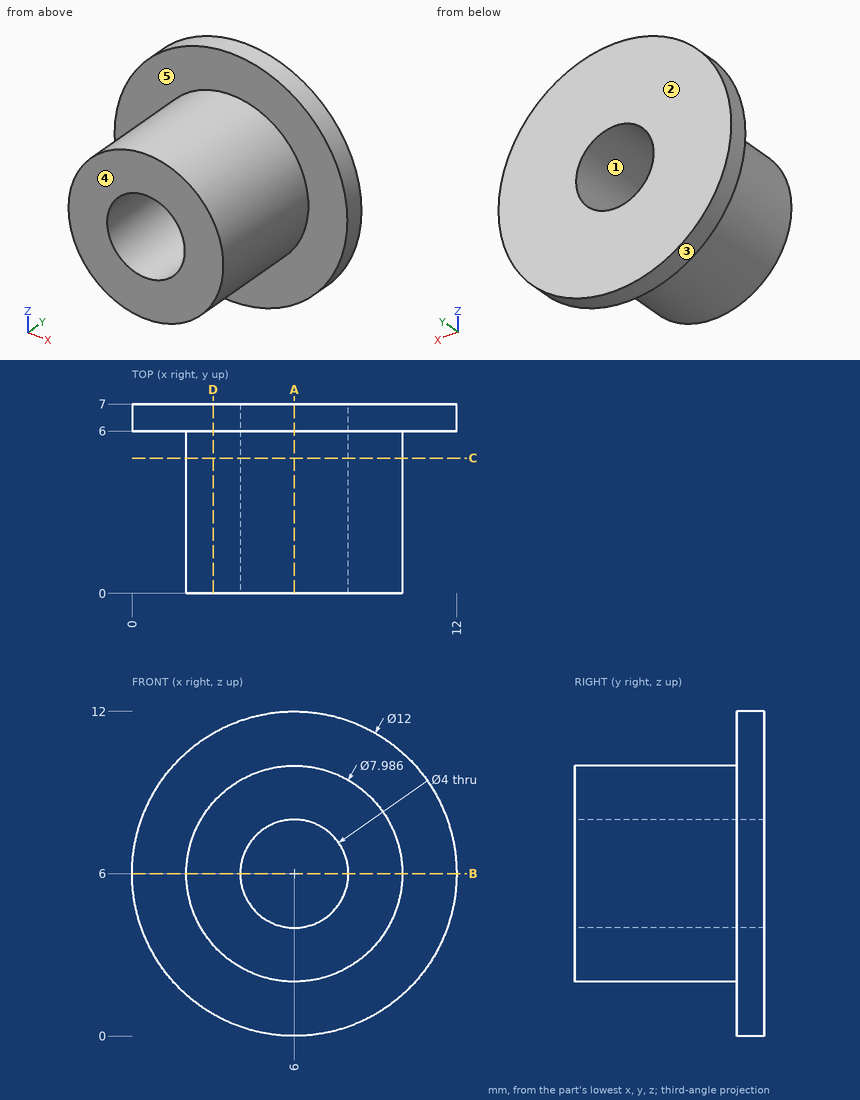
Verification items for this drawing (mm, ordinates from the low corner). A direction names the side the tool comes from. Coordinates: 2 decimals unless noted, no trailing zeros. Loops run counter-clockwise (first coordinate to the right, second up) from the corner with the lowest first, then second, coordinate; pieces in that order, holes last. Notation, with made-up numbers: (77.25, 82.5) -> (119.25, 82.5) arc R29 cw to (119.25, 116.5) -> close; hole circle Ø1 at (29.5, 84.25). An arc over 180 degrees is marked (long way). Answer in a Markdown table with one row per item. Add a question column.
1. Section check A-A, the plane x = 6. Enter the section's corners in (y, z), then the cut area to 3 significant figures.
2. Access from +Z, -Z, +X, -X, +Y, -Y to the whole of each face (thin tool, end or side, straight path). Record for the marked faces 4 and 5.
3. Section check C-C, the plane y = 5. Enter the section's corners in (x, z), then the cut area to 3 significant figures.
4. Section check D-D, the plane x = 3. Enter the section's corners in (y, z), then the cut area to 3 significant figures.
5. Material ranges on probe 1 along Z at (x, y) = (6, 4); probe 2 along Y at (x, z) = (10.75, 5.5); probe 3 along X at (y, z) = (4, 7.25), recorded low to high. Write a range as [from, to].
6. Draft check along Z on the marked faces 1, 2 and 3. Enter one of: +Z half, -Z half, draft (parallel to the pull), parting line (faces both ways), or undercut.
7. Section check B-B, the plane z = 6. Enter the section's corners in (x, y).
8. Depth check by flat-ended pin: P1, Ø3, axis at x = 1.5, y = 3.5, coming from the +Z side. Enter the tip coordinate at first touch or a pass-through.
Derived:
| question | item | result |
|---|---|---|
| 1 | outline | (0, 2.01) -> (6, 2.01) -> (6, 0) -> (7, 0) -> (7, 4) -> (0, 4) -> close; (0, 8) -> (7, 8) -> (7, 12) -> (6, 12) -> (6, 9.99) -> (0, 9.99) -> close |
| 1 | area | 31.9 mm² |
| 2 | face 4 | +Z, -Z, +X, -X, -Y |
| 2 | face 5 | -Y |
| 3 | outline | circle Ø7.99 at (6, 6); hole circle Ø4 at (6, 6) |
| 3 | area | 37.5 mm² |
| 4 | outline | (0, 3.36) -> (6, 3.36) -> (6, 0.8) -> (7, 0.8) -> (7, 11.2) -> (6, 11.2) -> (6, 8.64) -> (0, 8.64) -> close |
| 4 | area | 42.0 mm² |
| 5 | probe 1 | z = [2.01, 4], [8, 9.99] |
| 5 | probe 2 | y = [6, 7] |
| 5 | probe 3 | x = [2.21, 4.44], [7.56, 9.79] |
| 6 | face 1 | undercut |
| 6 | face 2 | draft |
| 6 | face 3 | parting line |
| 7 | outline | (0, 6) -> (2.01, 6) -> (2.01, 0) -> (4, 0) -> (4, 7) -> (0, 7) -> close; (8, 0) -> (9.99, 0) -> (9.99, 6) -> (12, 6) -> (12, 7) -> (8, 7) -> close |
| 8 | P1 | stops at z = 8.64 |
